Here's how the part is built. I have some questions about the finished solid (model axes, mm). A direction names the side the tool comes from. Coordinates: 2 decimals unless noted, no trailing zeros. Write each loop counter-clockwise with the first axis right and the second up, starting at its lowest first coordinate (ties: lowest second). Pieces come first, ordered by that corner, then holes.
```python
from build123d import *

# Parameters (mm, degrees)
BOSS_EXTRUDE1_DEPTH = 57.15
SKETCH4_W           = 21.391570407
SKETCH4_H           = 73.03
BOSS_EXTRUDE2_DEPTH = 4
SKETCH5_W           = 119.908429593
SKETCH5_H           = 73.03
BOSS_EXTRUDE3_DEPTH = 4


with BuildPart() as part:
    # Sketch3 → Boss-Extrude1 (new body)
    with BuildSketch(Plane(origin=(0, 0, 0), x_dir=(1, 0, 0), z_dir=(0, 1, 0))):
        with BuildLine():
            Line((-27.78125, 0), (-27.78125, 25.4))
            Line((-27.78125, 25.4), (-11.361506121, 25.4))
            ThreePointArc((-11.361506121, 25.4), (-9.864796768, 24.341666667), (-10.363699885, 22.577777778))
            ThreePointArc((-10.363699885, 22.577777778), (-15.08125, 12.7), (-10.363699885, 2.822222222))
            ThreePointArc((-10.363699885, 2.822222222), (-9.864796768, 1.058333333), (-11.361506121, 0))
            Line((-11.361506121, 0), (-27.78125, 0))
        make_face()
    extrude(amount=BOSS_EXTRUDE1_DEPTH)

    # Sketch4 → Boss-Extrude2 (add)
    with BuildSketch(Plane.XZ):
        with Locations((-17.085464796, -13.384999898)):
            Rectangle(SKETCH4_W, SKETCH4_H)
    extrude(amount=BOSS_EXTRUDE2_DEPTH)

    # Sketch5 → Boss-Extrude3 (add)
    with BuildSketch(Plane(origin=(0, -4, 0), x_dir=(-1, 0, 0), z_dir=(0, -1, 0))):
        with Locations((-53.564535204, 13.384999898)):
            Rectangle(SKETCH5_W, SKETCH5_H)
    extrude(amount=-BOSS_EXTRUDE3_DEPTH)


solid = part.part
```
1) Imagine slicing it at D-D on z = -36.5. Please give me the cut outline in (x, y).
Values follow:
outline: (-27.78, -4) - (113.52, -4) - (113.52, 0) - (-27.78, 0) - close
2) We'd pull the mould along Z, two halves only. Please class faces 4 (the face through (113.519, -2, -13)), 5 (the face through (-9.874, 28.175, -24.367)), 6 (the face through (-19, 28, 0)): pulls with the +Z half, pulls with the -Z half, needs draft (parallel to the pull), parting line crosses it, or undercut.
Values follow:
face 4: needs draft
face 5: undercut
face 6: pulls with the +Z half
3) Imagine slicing it at C-C on x = 2.5. Please give me the cut outline in (y, z), then the cut area to 3 significant figures.
Values follow:
outline: (-4, -49.9) - (0, -49.9) - (0, 23.13) - (-4, 23.13) - close
area: 292 mm2
4) I need wall thicknesses on probe 1 along Y at (x, z) = (61, -10); probe 2 along X at (y, z) = (5.5, -23.5); probe 3 along X at (y, z) = (49.5, -10). Which ranges of each line are inside material? Lowest first, please.
Values follow:
probe 1: y = -4 to 0
probe 2: x = -27.78 to -9.81
probe 3: x = -27.78 to -14.79
5) Imagine slicing it at B-B on z = -16. Please give me the cut outline in (x, y).
Values follow:
outline: (-27.78, -4) - (113.52, -4) - (113.52, 0) - (-14.65, 0) - (-14.65, 57.15) - (-27.78, 57.15) - close
6) On a 3-axis mill with a long thin cutter (end or side, diameter ignored), from which of +Z, -Z, +X, -X, +Y, -Y can I reach the whole of each face in a straight line? I mean faces 1 (the face through (-20, 28, -25.4)), 2 (the face through (-15.08, 28.17, -12.86)), 3 (the face through (44, -4, -14)). Say none if no direction works.
Values follow:
face 1: -Z, +X, -X, +Y
face 2: +X, +Y
face 3: +Z, -Z, +X, -X, -Y
7) Will these pins go through, and if not, where does the flat tip stop? pin 1 (18 mm diameter, centred on x = -21, y = 22.5, fed in from -Z); pin 2 (18 mm diameter, centred on x = -23.5, y = 29.5, fed in from +Z); pin 3 (10 mm diameter, centred on x = 58.5, z = -32, fed in from +Y).
Values follow:
pin 1: stops at z = -25.4
pin 2: stops at z = 0
pin 3: stops at y = 0
8) Imagine slicing it at A-A on y = 14.5. Please give me the cut outline in (x, z) (1 decimal), then the cut area to 3 significant figures.
Values follow:
outline: (-27.8, -25.4) - (-11.4, -25.4) arc R1.6 ccw to (-10.4, -22.6) arc R12.7 cw to (-10.4, -2.8) arc R1.6 ccw to (-11.4, 0) - (-27.8, 0) - close
area: 379 mm2
